from build123d import *

# Parameters (mm, degrees)
F1_DEPTH  = 7.5
F2_DEPTH  = 47
F3_W      = 98
F3_H      = 38
F3_H_2    = 303.1999886395
F4_DEPTH  = 1080
F5_W      = 303.1999886395
F5_H      = 552.5
F5_H_2    = 235
F6_DEPTH  = 1150.001
F7_DEPTH  = 1150
F8_W      = 954
F8_H      = 379.1999886395
F9_DEPTH  = 49
F5_H_3    = 162
F10_DEPTH = 1150
F11_W     = 303.1999886395
F11_H     = 162
F12_DEPTH = 10
F13_W     = 303.1999886395
F13_H     = 162
F14_DEPTH = 10
F5_H_4    = 15
F15_DEPTH = 1150


with BuildPart() as f1:
    # F0 (on Top) → F1 (new body, symmetric)
    with BuildSketch(Plane.XY):
        Polygon((550.5168708265, 71.7507553279), (574.5168708265, 96.5507666884), (513.4356752447, 155.6615740446), (490.2098794325, 131.6615740446), align=None)
        Polygon((513.4356752447, 155.6615740446), (-514.4019335917, 155.6615740446), (-491.1761377795, 131.6615740446), (490.2098794325, 131.6615740446), align=None)
        Polygon((-514.4019335917, 155.6615740446), (-575.4831291735, 96.5507666884), (-551.4831291735, 71.7507553279), (-491.1761377795, 131.6615740446), align=None)
        Polygon((-575.4831291735, 96.5507666884), (-575.4831291735, -331.4492333116), (-551.4831291735, -307.4492333116), (-551.4831291735, 71.7507553279), align=None)
        Polygon((550.5168708265, -307.4492333116), (574.5168708265, -331.4492333116), (574.5168708265, 96.5507666884), (550.5168708265, 71.7507553279), align=None)
        Polygon((-551.4831291735, -307.4492333116), (-575.4831291735, -331.4492333116), (574.5168708265, -331.4492333116), (550.5168708265, -307.4492333116), align=None)
        Polygon((-551.4831291735, 71.7507553279), (-551.4831291735, -307.4492333116), (550.5168708265, -307.4492333116), (550.5168708265, 71.7507553279), (490.2098794325, 131.6615740446), (-491.1761377795, 131.6615740446), align=None)
    extrude(amount=F1_DEPTH, both=True)

    # F0 (on Top) → F2 (join)
    with BuildSketch(Plane.XY):
        Polygon((-551.4831291735, -307.4492333116), (-575.4831291735, -331.4492333116), (574.5168708265, -331.4492333116), (550.5168708265, -307.4492333116), align=None)
        Polygon((-575.4831291735, 96.5507666884), (-575.4831291735, -331.4492333116), (-551.4831291735, -307.4492333116), (-551.4831291735, 71.7507553279), align=None)
        Polygon((550.5168708265, -307.4492333116), (574.5168708265, -331.4492333116), (574.5168708265, 96.5507666884), (550.5168708265, 71.7507553279), align=None)
        Polygon((-514.4019335917, 155.6615740446), (-575.4831291735, 96.5507666884), (-551.4831291735, 71.7507553279), (-491.1761377795, 131.6615740446), align=None)
        Polygon((550.5168708265, 71.7507553279), (574.5168708265, 96.5507666884), (513.4356752447, 155.6615740446), (490.2098794325, 131.6615740446), align=None)
        Polygon((513.4356752447, 155.6615740446), (-514.4019335917, 155.6615740446), (-491.1761377795, 131.6615740446), (490.2098794325, 131.6615740446), align=None)
    extrude(amount=F2_DEPTH)

    # F3 (on face) → F4 (join)
    with BuildSketch(Plane.XY.offset(7.5)):
        with Locations((-526.4831291735, -288.4492333116)):
            Rectangle(F3_W, F3_H)
        with Locations((-526.4831291735, -117.8492389919)):
            Rectangle(F3_W, F3_H_2)
        with Locations((-526.4831291735, 52.7507553279)):
            Rectangle(F3_W, F3_H)
        with Locations((525.5168708265, -288.4492333116)):
            Rectangle(F3_W, F3_H)
        with Locations((525.5168708265, -117.8492389919)):
            Rectangle(F3_W, F3_H_2)
        with Locations((525.5168708265, 52.7507553279)):
            Rectangle(F3_W, F3_H)
    extrude(amount=F4_DEPTH)

    # F5 (on face) → F6 (cut, through all)
    with BuildSketch(Plane(origin=(-575.4831291735, 0, 0), x_dir=(0, -1, 0), z_dir=(-1, 0, 0))):
        with Locations((117.8492389919, 811.25)):
            Rectangle(F5_W, F5_H)
        with Locations((117.8492389919, 364.5)):
            Rectangle(F5_W, F5_H_2)
    extrude(amount=-F6_DEPTH, mode=Mode.SUBTRACT)

    # F5 (on face) → F7 (join)
    with BuildSketch(Plane(origin=(-575.4831291735, 0, 0), x_dir=(0, -1, 0), z_dir=(-1, 0, 0))):
        Polygon((-71.7507553279, 1087.5), (-33.7507553279, 1087.5), (269.4492333116, 1087.5), (307.4492333116, 1087.5), (307.4492333116, 1125.5), (-71.7507553279, 1125.5), align=None)
    extrude(amount=-F7_DEPTH)

    # F8 (on face) → F9 (cut, symmetric)
    with BuildSketch(Plane.XY.offset(1125.5)):
        with Locations((-0.4831291735, -117.8492389919)):
            Rectangle(F8_W, F8_H)
    extrude(amount=F9_DEPTH, both=True, mode=Mode.SUBTRACT)

    # F5 (on face) → F10 (cut)
    with BuildSketch(Plane(origin=(-575.4831291735, 0, 0), x_dir=(0, -1, 0), z_dir=(-1, 0, 0))):
        with Locations((117.8492389919, 128)):
            Rectangle(F5_W, F5_H_3)
    extrude(amount=-F10_DEPTH, mode=Mode.SUBTRACT)

    # F11 (on face) → F12 (join)
    with BuildSketch(Plane.YZ.offset(-477.4831291735)):
        with Locations((-117.8492389919, 128)):
            Rectangle(F11_W, F11_H)
    extrude(amount=-F12_DEPTH)

    # F13 (on face) → F14 (join)
    with BuildSketch(Plane(origin=(476.5168708265, 0, 0), x_dir=(0, -1, 0), z_dir=(-1, 0, 0))):
        with Locations((117.8492389919, 128)):
            Rectangle(F13_W, F13_H)
    extrude(amount=-F14_DEPTH)

    # F5 (on face) → F15 (join)
    with BuildSketch(Plane(origin=(-575.4831291735, 0, 0), x_dir=(0, -1, 0), z_dir=(-1, 0, 0))):
        with Locations((117.8492389919, 489.5)):
            Rectangle(F5_W, F5_H_4)
    extrude(amount=-F15_DEPTH)


solid = f1.part
The model under review builds one solid part; all positions refer to its coordinate system, in mm. A direction names the side the tool comes from. Coordinates: 2 decimals unless noted, no trailing zeros. Loops run counter-clockwise (first coordinate to the right, second up) from the corner with the lowest first, then second, coordinate; pieces in that order, holes last. Notation, with made-up numbers: M -9,-29.5 L 22,-29.5 A7 ccw 22,-21.5 Z; hole C 38,6.25 d1. An arc over 180 degrees is marked long. Put each result on its own line as item: value. Start each with the question number.
Q1. Wall thickness on line 1 (Y direction, x = 497.5, z = 792); line 2 (Z direction, x = -125.5, y = -60); line 3 (X direction, y = -156.5, z = 146): over which ranges is each line inside the solid? List them lowest first.
Q2. The part is to be moulded in two halves that separate along Y. For faces 1 (the flat face through (544.404, 125.692, 19.368)), 2 (the flat face through (525, -121, 1125.5)), 3 (the flat face through (-527, -116, 535)), say which applies: +Y half, -Y half, draft (parallel to the pull), parting line (faces both ways), or undercut.
Q3. Add section C-C (z = 1019.5). Write out the cut boundary in (x, y), and give its area (3 significant figures).
Q4. Add section B-B (x = -301.5). Write out the cut boundary in (y, z), and give its area (3 significant figures).
Q5. For faces 4 (the flat face through (-9, 142, 47)), 5 (the flat face through (525, 33.751, 363)), 6 (the flat face through (530, -116, 209)), 7 (the flat face through (-532, 33.751, 127)), 8 (the flat face through (525, -307.449, 579)), list the 3-axis set-ups (+Z, -Z, +X, -X, +Y, -Y) from which the entire face can be reached by the end or side of a thin tool; tool diameter is ignored.
Q6. Add section A-A (y = -228). Count the separate pieces of the cut face and the enclosed holes in it, and give its area (3 significant figures).
Q7. Clearance check with flat-ended pins moving along their axes: pin 1 (4 mm diameter, centred on y = -236.5, z = 106, fed in from +X); pin 2 (4 mm diameter, centred on x = 222.5, y = -65.5, fed in from +Z); pin 3 (10 mm diameter, centred on x = 217, y = 70, fed in from +Z). State where each tip first meets the part, or that it passes through.
Answers:
1. line 1: y = -307.45 to -269.45, 33.75 to 71.75
1. line 2: z = -7.5 to 7.5, 482 to 497
1. line 3: x = -487.48 to -477.48, 476.52 to 486.52
2. face 1: +Y half
2. face 2: draft
2. face 3: undercut
3. outline: M -575.48,-307.45 L -477.48,-307.45 L -477.48,-269.45 L -575.48,-269.45 Z; M -575.48,33.75 L -477.48,33.75 L -477.48,71.75 L -575.48,71.75 Z; M 476.52,-307.45 L 574.52,-307.45 L 574.52,-269.45 L 476.52,-269.45 Z; M 476.52,33.75 L 574.52,33.75 L 574.52,71.75 L 476.52,71.75 Z
3. area: 14,900 mm^2
4. outline: M -331.45,-7.5 L 155.66,-7.5 L 155.66,47 L 131.66,47 L 131.66,7.5 L -307.45,7.5 L -307.45,47 L -331.45,47 Z; M -269.45,482 L 33.75,482 L 33.75,497 L -269.45,497 Z
4. area: 13,800 mm^2
5. face 4: +Z, +X, -X, +Y
5. face 5: +X, -X
5. face 6: +X
5. face 7: -X
5. face 8: +Z, +X, -X, -Y
6. separate pieces: 4
6. enclosed holes: 0
6. area: 67,800 mm^2
7. pin 1: stops at x = 486.52
7. pin 2: stops at z = 497
7. pin 3: stops at z = 7.5
